The model under review builds one solid part; all positions refer to its coordinate system, in mm. Round coordinates to 2 decimals unless told otherwise and drop trailing zeros. Loops run counter-clockwise (first coordinate to the right, second up) from the corner with the lowest first, then second, coordinate; pieces in that order, holes last. Notation, with made-up numbers: M 38,51.5 L 94,51.5 A16 cw 94,69.5 Z; hole C 37,33 d3. An arc over 180 degrees is marked long. Answer as a JSON object with one key per item and string values. Group by question number.
Item 1: Consider section B-B (x = 0.1). Give the boundary of the cut face in (y, z).
Item 2: Consider section A-A (z = 0.1). Give the boundary of the cut face in (x, y), and give its area (3 significant figures).
Item 3: To check wall thickness, follow line 1 (Y direction, x = 0.25, z = 0.1); line 2 (Y direction, x = 0.5, z = 0.6). State the ranges of each line that lie inside material, in increasing order.
```python
from build123d import *

# Parameters (mm, degrees)
PIN_DRAWING_W = 0.636
PIN_DRAWING_H = 0.636
PIN_DEPTH     = 11.54
CHAMFER2_SIZE = 0.2


with BuildPart() as part:
    # pin_drawing → pin (new body)
    with BuildSketch(Plane(origin=(0, 0, 0), x_dir=(1, 0, 0), z_dir=(0, 1, 0))):
        with Locations((0.318, -0.318)):
            Rectangle(PIN_DRAWING_W, PIN_DRAWING_H)
    extrude(amount=PIN_DEPTH)

    # Chamfer2
    chamfer2_edges = [part.edges().sort_by_distance(p)[0] for p in [
        (0.636, 11.54, 0.318),
        (0.318, 11.54, 0),
        (0, 11.54, 0.318),
        (0.318, 0, 0),
        (0.636, 0, 0.318),
        (0.318, 0, 0.636),
        (0, 0, 0.318),
        (0.318, 11.54, 0.636),
    ]]
    chamfer(chamfer2_edges, length=CHAMFER2_SIZE)


solid = part.part
```
Geometry results:
{
 "1": {"outline": "M 0.1,0.1 L 0.2,0 L 11.34,0 L 11.44,0.1 L 11.44,0.54 L 11.34,0.64 L 0.2,0.64 L 0.1,0.54 Z"},
 "2": {"outline": "M 0,0.2 L 0.1,0.1 L 0.54,0.1 L 0.64,0.2 L 0.64,11.34 L 0.54,11.44 L 0.1,11.44 L 0,11.34 Z", "area": "7.19 mm^2"},
 "3": {"line 1": "y = 0.1 to 11.44", "line 2": "y = 0.16 to 11.38"}
}
